from build123d import *

# Parameters (mm, degrees)
F0_W     = 125
F0_H     = 28
F1_DEPTH = 8
F2_R     = 13.99999
F3_SIZE  = 0.6


# Not quite as in the source:
# - a fillet or chamfer is up to 0.001 mm smaller than in the source, because OpenCascade refuses the exact size


with BuildPart() as f1:
    # F0 (on Front) → F1 (new body, symmetric)
    with BuildSketch(Plane.XZ):
        Rectangle(F0_W, F0_H)
    extrude(amount=F1_DEPTH, both=True)

    # F2 (radius 14 in the source; OpenCascade refuses exactly that, so slightly less here)
    f2_edges = [f1.edges().sort_by_distance(p)[0] for p in [
        (62.5, 0, -14),
        (62.5, 0, 14),
        (-62.5, 0, -14),
        (-62.5, 0, 14),
    ]]
    fillet(f2_edges, radius=F2_R)

    # F3
    f3_edges = [f1.edges().sort_by_distance(p)[0] for p in [
        (0, -8, 14),
        (62.5, -8, 0),
        (58.399498, -8, -9.899498),
        (58.399498, -8, 9.899498),
        (0, -8, -14),
        (-58.399498, -8, -9.899498),
        (-58.399498, -8, 9.899498),
        (-62.5, -8, 0),
        (62.5, 8, 0),
        (58.399498, 8, -9.899498),
        (58.399498, 8, 9.899498),
        (0, 8, -14),
        (0, 8, 14),
        (-58.399498, 8, -9.899498),
        (-58.399498, 8, 9.899498),
        (-62.5, 8, 0),
    ]]
    chamfer(f3_edges, length=F3_SIZE)


solid = f1.part
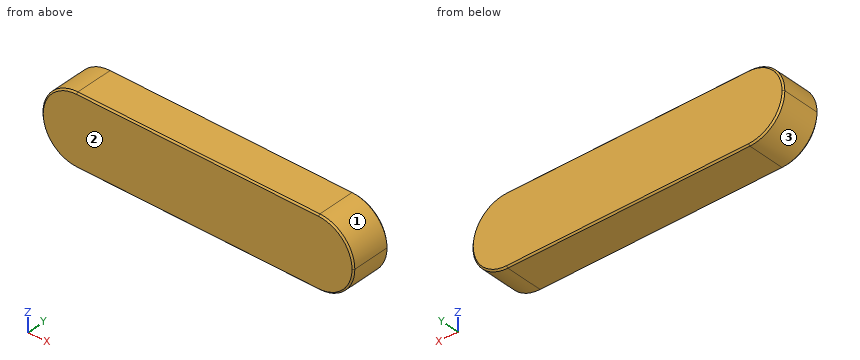
Here's how the part is built. I have some questions about the finished solid (model axes, mm). Face numbers are marked on the shaded views. Round coordinates to 2 decimals unless told otherwise and drop trailing zeros. One line per question, with ' | ' between items.
1) I'm going to push flat-ended pins straight in: pin 1 Ø8 at (y, z) = (0, 5.5) entering from +X; pin 2 Ø5 at (y, z) = (1, 9) entering from +X. Where does each tip first touch, or does it pass through?
Checked values:
pin 1: stops at x = 62.42 | pin 2: stops at x = 60.9
2) We'd pull the mould along Z, two halves only. Please class the marked faces 1, 2 and 3: released by +Z, released by -Z, zero draft, split by the parting line, or undercut.
Checked values:
face 1: released by +Z | face 2: zero draft | face 3: released by -Z
3) I need wall thicknesses on line 1 (Z direction, x = -57, y = 4); line 2 (Z direction, x = 52.5, y = 6.5); line 3 (X direction, y = -5.5, z = -7). Which ranges of each line are inside material? Lowest first, please.
Checked values:
line 1: z = -11.12 to 11.12 | line 2: z = -13.42 to 13.42 | line 3: x = -60.62 to 60.62
